from build123d import *

# Parameters (mm, degrees)
F0_R     = 9
F0_R_2   = 6
F1_DEPTH = 2.5
F0_R_3   = 10.75
F0_R_4   = 4
F2_DEPTH = 3.5
F4_SIZE  = 0.9


with BuildPart() as f1:
    # F0 (on Top) → F1 (new body, symmetric)
    with BuildSketch(Plane.XY):
        Circle(F0_R)
        Circle(F0_R_2, mode=Mode.SUBTRACT)
    extrude(amount=F1_DEPTH, both=True)

    # F0 (on Top) → F2 (join, symmetric)
    with BuildSketch(Plane.XY):
        Circle(F0_R_3)
        Circle(F0_R, mode=Mode.SUBTRACT)
        Circle(F0_R_2)
        Circle(F0_R_4, mode=Mode.SUBTRACT)
    extrude(amount=F2_DEPTH, both=True)


with BuildPart() as f1_1:
    # F3: moved
    add(f1.part.moved(Location((0, 0, 4.5))))

    # F4
    f4_edges = [f1_1.edges().sort_by_distance(p)[0] for p in [
        (-4, 0, 8),
        (-4, 0, 1),
    ]]
    chamfer(f4_edges, length=F4_SIZE)


with BuildPart() as f1_2:
    # F5: moved
    add(f1_1.part.moved(Location((0, 0, 2.5))))


solid = f1_2.part
Build history of the part. All positions in model axes, mm. A direction names the side the tool comes from. Coordinates: 2 decimals unless noted, no trailing zeros. Order: outer loops, then holes, each group sorted by start corner. A loop starts at its lowest first (then second) coordinate and runs counter-clockwise, first axis right, second up. Notation, with made-up numbers: (-19.75, 46.25) - (13.25, 46.25) arc R17 ccw to (13.25, 52.25) - close; hole circle Ø4 at (72.25, 14). An arc over 180 degrees is marked (long way). Put each result on its own line as item: value.
1. Probe line 1 along Y through (x, z) = (-3.5, 4.25); line 2 along Y through (x, z) = (0, 4.05); line 3 along X through (y, z) = (-1.75, 5.25). List the from-to ranges inside material, lowest first. Write a range as [from, to].
Answer sheet:
line 1: y = [-10.16, -8.29], [-4.87, -2.23], [2.23, 4.87], [8.29, 10.16]
line 2: y = [-10.75, -9], [-6, -4.35], [4.35, 6], [9, 10.75]
line 3: x = [-10.61, -3.6], [3.6, 10.61]
2. Drop flat-ended pins along their axis: P1, Ø1.5, axis at x = -8.5, z = 5, coming from the +Y side; P2, Ø2, axis at x = 8, z = 9, coming from the -Y side; P3, Ø1, axis at x = -8, z = 6.5, coming from the -Y side. Give the stop position or say it passes through.
Answer sheet:
P1: stops at y = 7.45
P2: stops at y = -8.16
P3: stops at y = -7.7
3. Saw through at D-D (y = 8.25). Write the cut outline in (x, z), and give its area (3 significant figures).
Answer sheet:
outline: (-6.89, 3.5) - (-3.6, 3.5) - (-3.6, 4.5) - (3.6, 4.5) - (3.6, 3.5) - (6.89, 3.5) - (6.89, 10.5) - (3.6, 10.5) - (3.6, 9.5) - (-3.6, 9.5) - (-3.6, 10.5) - (-6.89, 10.5) - close
area: 82.1 mm^2
4. Pull direction Y, two halves, no side cores. Call faces 1 (the face through (-0.867, -3.905, 6.964)), 2 (the face through (-1.4, 10.66, 7.05)), 3 (the face through (1, -5, 3.5)): pulls with the +Y half, pulls with the -Y half, needs draft (parallel to the pull), parting line crosses it, or undercut.
Answer sheet:
face 1: undercut
face 2: parting line crosses it
face 3: needs draft
5. Saw through at B-B (z = 10). Write the cut outline in (x, y).
Answer sheet:
outline: circle Ø21.5 at (0, 0); circle Ø12 at (0, 0); hole circle Ø18 at (0, 0); hole circle Ø8.8 at (0, 0)
6. Tool access for faces 4 (the face through (-1.172, 8.923, 9.993)), 5 (the face through (2, -6, 4.5)), 6 (the face through (-2, -9, 10.5)): list every direction of +Z, -Z, +X, -X, +Y, -Y with a clear straight run to the whole face (end or side of a thin tool).
Answer sheet:
face 4: +Z
face 5: -Z
face 6: +Z, +X, -X, +Y, -Y
7. Saw through at A-A (x = 0). Write the cut outline in (y, z).
Answer sheet:
outline: (-10.75, 3.5) - (-9, 3.5) - (-9, 4.5) - (-6, 4.5) - (-6, 3.5) - (-4.9, 3.5) - (-4, 4.4) - (-4, 9.6) - (-4.9, 10.5) - (-6, 10.5) - (-6, 9.5) - (-9, 9.5) - (-9, 10.5) - (-10.75, 10.5) - close; (4, 4.4) - (4.9, 3.5) - (6, 3.5) - (6, 4.5) - (9, 4.5) - (9, 3.5) - (10.75, 3.5) - (10.75, 10.5) - (9, 10.5) - (9, 9.5) - (6, 9.5) - (6, 10.5) - (4.9, 10.5) - (4, 9.6) - close
